Autodesk Inventor part; units mm, degrees
ref_plane "YZ Plane" through (0, 0, 0) normal (1, 0, 0) x (0, 1, 0)
ref_plane "XZ Plane" through (0, 0, 0) normal (0, 1, 0) x (-1, 0, 0)
ref_plane "XY Plane" through (0, 0, 0) normal (0, 0, 1) x (1, 0, 0)
sketch "草图1" plane through (0, 0, 0) normal (0, 0, 1) x (1, 0, 0)
  circle A0 centre (0, 0) radius 70
  dimension "d0" = 140
extrude "拉伸1" add sketch "草图1" along normal blind 8
sketch "草图2" plane through (0, 0, 0) normal (0, 0, -1) x (-1, 0, 0)
  circle A0 centre (0, 0) radius 40
  circle A1 centre (0, 0) radius 30
  dimension "d3" = 80
  dimension "d4" = 60
extrude "拉伸2" add sketch "草图2" along normal blind 12
sketch "草图3" plane through (0, 0, -12) normal (0, 0, -1) x (-1, 0, 0)
  circle A0 centre (0, 0) radius 40
  circle A1 centre (0, 0) radius 39
  dimension "d7" = 80
  dimension "d8" = 78
extrude "拉伸3" cut sketch "草图3" against normal blind 4
fillet "圆角2" radius 1 1 edges at (-70, 0, 8)
sketch "草图5" plane through (0, 0, 8) normal (0, 0, 1) x (1, 0, 0)
  circle A0 centre (-55, 0) radius 4
  line L0 (0, 0) -> (-8.161, 0)
  dimension "d16" = 8
  dimension "d17" = 8.161
  dimension "d18" = 55
extrude "拉伸5" cut sketch "草图5" against normal through all
pattern_circular "环形阵列1" count 6 over 360 about axis through (0, 0, -10) along (0, 0, 1) of "拉伸5"
sketch "草图6" plane through (0, 0, 8) normal (0, 0, 1) x (1, 0, 0)
  circle A0 centre (0, 0) radius 40
  dimension "d24" = 80
extrude "拉伸6" add sketch "草图6" along normal blind 6
sketch "草图7" plane through (0, 0, 14) normal (0, 0, 1) x (1, 0, 0)
  circle A0 centre (0, 0) radius 20.5
  dimension "d27" = 41
extrude "拉伸7" cut sketch "草图7" against normal through all
fillet "圆角3" radius 3 2 edges at (-40, 0, 14) (-40, 0, 8)
properties part number "主动轴大端盖"
Design review of the part built by this model. Coordinates are the model's own, in mm. A direction names the side the tool comes from. Give positions to 0.01 mm unless a question says otherwise; leave off trailing zeros. Order: outer loops, then holes, each group sorted by start corner. A loop starts at its lowest first (then second) coordinate and runs counter-clockwise, first axis right, second up. Notation, with made-up numbers: (-32, -33) - (21, -33) arc R18 cw to (21, -11) - close; hole circle Ø1 at (21.25, 62.25). An arc over 180 degrees is marked (long way). Write item = value, one per line. Start each with the question number.
Q1. Clearance check with flat-ended pins moving along their axes: pin 1 Ø6 at (x, z) = (-40, -7) entering from -Y; pin 2 Ø9 at (x, y) = (27.5, 47.63) entering from +Z; pin 3 Ø10 at (x, z) = (-1, 5.5) entering from +Y. State where each tip first meets the part, or that it passes through.
Q2. Tool access review of faces 4 (the face through (-20, -23, -12)), 5 (the face through (30, -30, 0)), 6 (the face through (-32, -30, 8)): name each direction out of +Z, -Z, +X, -X, +Y, -Y from which nothing blocks a thin tool from reaching the whole face with its end or side.
Q3. We need section B-B on y = 0. State how many separate pieces and enclosed holes the cut face has, plus the area to 3 significant figures.
Q4. Mouldability with a two-part tool opening along X and no side actions: class faces 1 (the face through (-55.55, 42.594, 3.451)), 2 (the face through (-51.185, 1.201, 4.056)), 3 (the face through (16, -16, 14)) as released by +X, released by -X, zero draft, split by the parting line, or undercut.
Q5. We need section C-C on z = -2. State the section outline as (x, y) points.
Q6. To check wall thickness, follow L1, parallel to Y at x = 0, z = 4.75; L2, parallel to Y at x = 27.5, z = 4; L3, parallel to Y at x = 0, z = 10.5. State the ranges of each line that lie inside material, in increasing order. Write a range as from..to.
Working result:
q1.pin_1 = -15.2
q1.pin_2 = 8
q1.pin_3 = 70
q2.face_4 = -Z, +X, -X, +Y, -Y
q2.face_5 = -Z
q2.face_6 = +Z
q3.separate_pieces = 4
q3.enclosed_holes = 0
q3.area = 1,130 mm²
q4.face_1 = split by the parting line
q4.face_2 = undercut
q4.face_3 = zero draft
q5.outline = circle Ø80 at (0, 0); hole circle Ø60 at (0, 0)
q6.L1 = -70..-20.5, 20.5..70
q6.L2 = -64.37..-51.63, -43.63..43.63, 51.63..64.37
q6.L3 = -40.04..-20.5, 20.5..40.04
